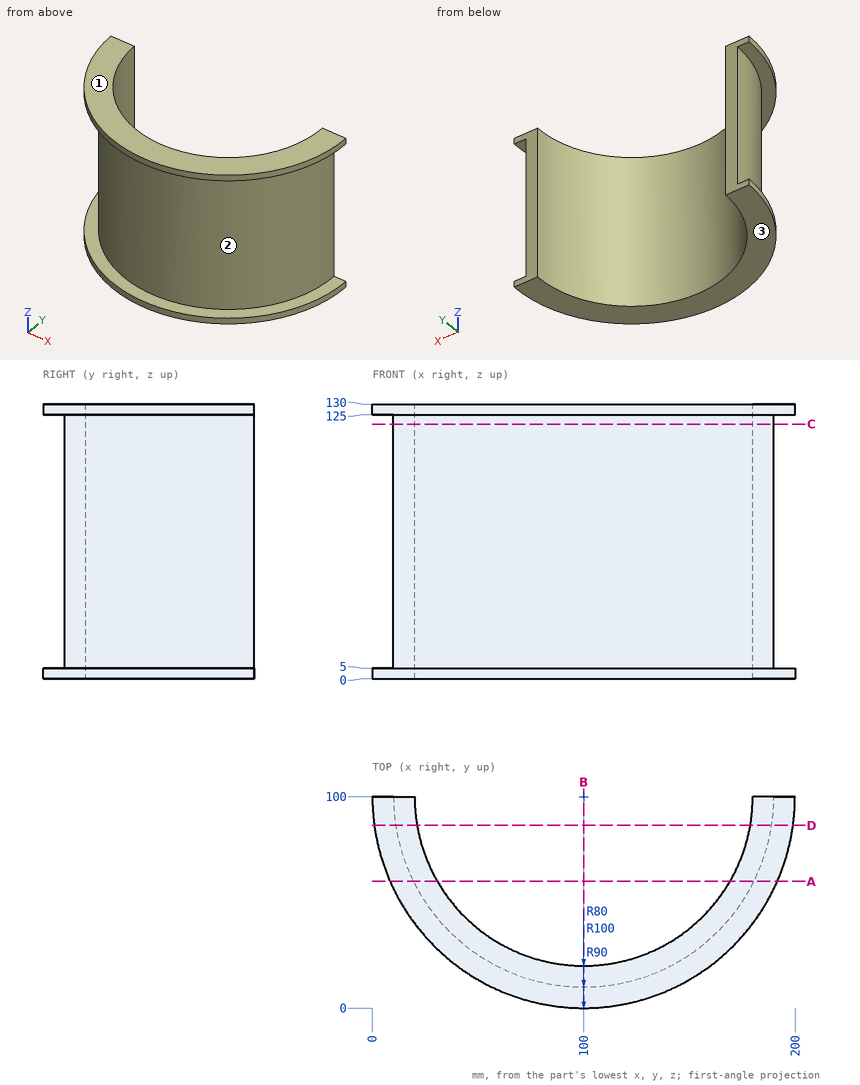
The figure shows three views and two pictorial views of one solid part (mm, origin at its lowest corner). Answer the questions. Coordinates: 2 decimals unless noted, no trailing zeros. Write each loop counter-clockwise with the first axis right and the second up, starting at its lowest first coordinate (ties: lowest second). Pieces come first, ordered by that corner, then holes. Notation, with made-up numbers: M 27.25,-2.5 L 39.25,-2.5 A20 ccw 39.25,6.5 Z; hole C 81.5,73 d9. An arc over 180 degrees is marked long. Answer as CSV lines item,"result". Start each with the question number.
Item 1: Section D-D on y = 86.5 is taken. Write down the section's boundary in (x, z), and give its area (3 significant figures).
Item 2: Section B-B on x = 100 is taken. Write down the section's boundary in (y, z), and give its area (3 significant figures).
Item 3: Section A-A on y = 60 is taken. Write down the section's boundary in (x, z).
Item 4: Determine the mould class of the marked faces 1, 2 and 3 for opening direction Z: released by +Z, released by -Z, zero draft, split by the parting line, or undercut.
Item 5: Section C-C on z = 120.5 is taken. Write down the section's boundary in (x, y), and give its area (3 significant figures).
Item 6: Flat-ended cylindrical pins translate along their axes: P1, Ø5, axis at y = 25.5, z = 76, coming from the +X side; P2, Ø1, axis at y = 58.5, z = 35.5, coming from the +X side; P3, Ø4, axis at x = 74.5, z = 19, coming from the +Y side; P4, Ø3, axis at x = 76.5, y = 26.5, coming from the +Z side. Find the tip coordinate at first contact, or state that the pin passes through.
Item 7: Consider L1, parallel to Z at x = 158, y = 26; L2, parallel to X at y = 43.5, z = 74.5; L3, parallel to X at y = 81, z = 16. Determine where each line is inside the solid, lowest interval first.
Checks:
1,outline,"M 0.92,0 L 21.15,0 L 21.15,130 L 0.92,130 L 0.92,125 L 11.02,125 L 11.02,5 L 0.92,5 Z; M 178.85,0 L 199.08,0 L 199.08,5 L 188.98,5 L 188.98,125 L 199.08,125 L 199.08,130 L 178.85,130 Z"
1,area,"2,840 mm²"
2,outline,"M 0,0 L 20,0 L 20,130 L 0,130 L 0,125 L 10,125 L 10,5 L 0,5 Z"
2,area,"1,400 mm²"
3,outline,"M 8.35,0 L 30.72,0 L 30.72,130 L 8.35,130 L 8.35,125 L 19.38,125 L 19.38,5 L 8.35,5 Z; M 169.28,0 L 191.65,0 L 191.65,5 L 180.62,5 L 180.62,125 L 191.65,125 L 191.65,130 L 169.28,130 Z"
4,face 1,"released by +Z"
4,face 2,"undercut"
4,face 3,"released by -Z"
5,outline,"M 10,100 A90 ccw 190,100 L 180,100 A80 cw 20,100 Z"
5,area,"2,670 mm²"
6,P1,"stops at x = 154"
6,P2,"stops at x = 180.12"
6,P3,"stops at y = 24.88"
6,P4,"passes through"
7,L1,"z = 0 to 5, 125 to 130"
7,L2,"x = 29.94 to 43.36, 156.64 to 170.06"
7,L3,"x = 12.03 to 22.29, 177.71 to 187.97"
